Design review of the part built by this model. Coordinates are the model's own, in mm. A direction names the side the tool comes from. Coordinates: 2 decimals unless noted, no trailing zeros. Loops run counter-clockwise (first coordinate to the right, second up) from the corner with the lowest first, then second, coordinate; pieces in that order, holes last. Notation, with made-up numbers: (27, -15) - (62, -15) arc R15 ccw to (62, -4) - close; hole circle Ø10 at (-4.5, 44). An arc over 180 degrees is marked (long way). One line per question, with ' | ' between items.
from build123d import *

# Parameters (mm, degrees)
BOSS_EXTRUDE1_DEPTH  = 58.71
SKETCH4_R            = 4.8
CUT_EXTRUDE1_DEPTH   = 1
SKETCH5_R            = 4.8
CUT_EXTRUDE2_DEPTH   = 1
SKETCH6_W            = 19
SKETCH6_H            = 26
BOSS_EXTRUDE3_DEPTH  = 58.71
SKETCH7_W            = 58.71
SKETCH7_H            = 17
SKETCH7_H_2          = 19
BOSS_EXTRUDE4_DEPTH  = 57
BOSS_EXTRUDE5_DEPTH  = 3
CUT_EXTRUDE3_DEPTH   = 17
CUT_EXTRUDE4_START   = -19
CUT_EXTRUDE4_DEPTH   = 19
CUT_EXTRUDE5_DEPTH   = 4.632332886
SKETCH12_W           = 5
SKETCH12_H           = 5
BOSS_EXTRUDE6_DEPTH  = 100
CHAMFER1_SIZE        = 3
SKETCH13_W           = 61.71
SKETCH13_H           = 17.5
BOSS_EXTRUDE7_DEPTH  = 17
SKETCH14_W           = 24.98
SKETCH14_H           = 2.38
SKETCH14_W_2         = 14.02
BOSS_EXTRUDE8_DEPTH  = 12.5
BOSS_EXTRUDE9_DEPTH  = 5
BOSS_EXTRUDE10_START = -5
BOSS_EXTRUDE10_DEPTH = 5


with BuildPart() as part:
    # Sketch3 → Boss-Extrude1 (new body)
    with BuildSketch(Plane.YZ):
        Polygon((0, 5), (0, 0), (17, 0), (81, 26), (100, 26), (100, 31), (81, 31), (17, 5), align=None)
    extrude(amount=BOSS_EXTRUDE1_DEPTH)

    # Sketch4 → Cut-Extrude1 (cut)
    with BuildSketch(Plane.XY.offset(31)):
        with Locations((12.75, 90.5)):
            Circle(SKETCH4_R)
        with Locations((47.2, 90.5)):
            Circle(SKETCH4_R)
    extrude(amount=-CUT_EXTRUDE1_DEPTH, mode=Mode.SUBTRACT)

    # Sketch5 → Cut-Extrude2 (cut)
    with BuildSketch(Plane.XY.offset(5)):
        with Locations((21.94, 8.5)):
            Circle(SKETCH5_R)
        with Locations((36.94, 8.5)):
            Circle(SKETCH5_R)
    extrude(amount=-CUT_EXTRUDE2_DEPTH, mode=Mode.SUBTRACT)

    # Sketch6 → Boss-Extrude3 (add)
    with BuildSketch(Plane.YZ.offset(58.71)):
        with Locations((90.5, 13)):
            Rectangle(SKETCH6_W, SKETCH6_H)
    extrude(amount=-BOSS_EXTRUDE3_DEPTH)

    # Sketch7 → Boss-Extrude4 (add)
    with BuildSketch(Plane(origin=(0, 0, 0), x_dir=(1, 0, 0), z_dir=(0, 0, -1))):
        with Locations((29.355, -8.5)):
            Rectangle(SKETCH7_W, SKETCH7_H)
        with Locations((29.355, -90.5)):
            Rectangle(SKETCH7_W, SKETCH7_H_2)
    extrude(amount=BOSS_EXTRUDE4_DEPTH)

    # Sketch8 → Boss-Extrude5 (add)
    with BuildSketch(Plane.YZ.offset(58.71)):
        Polygon((100, 31), (81, 31), (17, 5), (0, 5), (0, -57), (17, -57), (17, 0), (81, 26), (81, -57), (100, -57), align=None)
    extrude(amount=BOSS_EXTRUDE5_DEPTH)

    # Sketch9 → Cut-Extrude3 (cut)
    with BuildSketch(Plane.XZ):
        with BuildLine():
            Line((15, -2.5), (46.71, -2.5))
            ThreePointArc((46.71, -2.5), (53.781067812, -5.428932188), (56.71, -12.5))
            Line((56.71, -12.5), (56.71, -42))
            ThreePointArc((56.71, -42), (53.781067812, -49.071067812), (46.71, -52))
            Line((46.71, -52), (15, -52))
            ThreePointArc((15, -52), (7.928932188, -49.071067812), (5, -42))
            Line((5, -42), (5, -12.5))
            ThreePointArc((5, -12.5), (7.928932188, -5.428932188), (15, -2.5))
        make_face()
    extrude(amount=-CUT_EXTRUDE3_DEPTH, mode=Mode.SUBTRACT)

    # Sketch10 → Cut-Extrude4 (cut)
    with BuildSketch(Plane(origin=(0, 100, 0), x_dir=(-1, 0, 0), z_dir=(0, 1, 0)).offset(CUT_EXTRUDE4_START)):
        with BuildLine():
            Line((-46.71, 23.5), (-15, 23.5))
            ThreePointArc((-15, 23.5), (-7.928932188, 20.571067812), (-5, 13.5))
            Line((-5, 13.5), (-5, -42))
            ThreePointArc((-5, -42), (-7.928932188, -49.071067812), (-15, -52))
            Line((-15, -52), (-46.71, -52))
            ThreePointArc((-46.71, -52), (-53.781067812, -49.071067812), (-56.71, -42))
            Line((-56.71, -42), (-56.71, 13.5))
            ThreePointArc((-56.71, 13.5), (-53.781067812, 20.571067812), (-46.71, 23.5))
        make_face()
    extrude(amount=CUT_EXTRUDE4_DEPTH, mode=Mode.SUBTRACT)

    # Sketch11 → Cut-Extrude5 (cut)
    with BuildSketch(Plane(origin=(0, 0.664710813, -1.636211232), x_dir=(1, 0, 0), z_dir=(0, -0.376377046955938, 0.9264665771223093))):
        with BuildLine():
            Line((17, 79.711481203), (44.71, 79.711481203))
            ThreePointArc((44.71, 79.711481203), (51.781067812, 76.782549014), (54.71, 69.711481203))
            Line((54.71, 69.711481203), (54.71, 34.631817046))
            ThreePointArc((54.71, 34.631817046), (51.781067812, 27.560749234), (44.71, 24.631817046))
            Line((44.71, 24.631817046), (17, 24.631817046))
            ThreePointArc((17, 24.631817046), (9.928932188, 27.560749234), (7, 34.631817046))
            Line((7, 34.631817046), (7, 69.711481203))
            ThreePointArc((7, 69.711481203), (9.928932188, 76.782549014), (17, 79.711481203))
        make_face()
    extrude(amount=-CUT_EXTRUDE5_DEPTH, mode=Mode.SUBTRACT)

    # Sketch12 → Boss-Extrude6 (add)
    with BuildSketch(Plane.XZ):
        with Locations((2.5, -54.5)):
            Rectangle(SKETCH12_W, SKETCH12_H)
        with Locations((59.21, -54.5)):
            Rectangle(SKETCH12_W, SKETCH12_H)
    extrude(amount=-BOSS_EXTRUDE6_DEPTH)

    # Chamfer1
    chamfer1_edges = [part.edges().sort_by_distance(p)[0] for p in [
        (2.5, 17, -52),
        (2.5, 81, -52),
        (59.21, 81, -52),
        (59.21, 17, -52),
    ]]
    chamfer(chamfer1_edges, length=CHAMFER1_SIZE)

    # Sketch13 → Boss-Extrude7 (add)
    with BuildSketch(Plane.XZ):
        with Locations((30.855, -3.75)):
            Rectangle(SKETCH13_W, SKETCH13_H)
    extrude(amount=-BOSS_EXTRUDE7_DEPTH)

    # Sketch14 → Boss-Extrude8 (add)
    with BuildSketch(Plane.XZ):
        with Locations((12.49, -11.31)):
            Rectangle(SKETCH14_W, SKETCH14_H)
        with Locations((54.7, -11.31)):
            Rectangle(SKETCH14_W_2, SKETCH14_H)
    extrude(amount=BOSS_EXTRUDE8_DEPTH)

    # Sketch15 → Boss-Extrude9 (add)
    with BuildSketch(Plane(origin=(0, 0, 0), x_dir=(0, -1, 0), z_dir=(-1, 0, 0))):
        with BuildLine():
            Line((0, -12.5), (12.5, -12.5))
            ThreePointArc((12.5, -12.5), (4.446217859, -15.360002914), (0, -22.6589186))
            Line((0, -22.6589186), (0, -12.5))
        make_face()
    extrude(amount=-BOSS_EXTRUDE9_DEPTH)

    # Sketch16 → Boss-Extrude10 (add)
    with BuildSketch(Plane.YZ.offset(61.71).offset(BOSS_EXTRUDE10_START)):
        with BuildLine():
            Line((-12.5, -12.5), (0, -12.5))
            Line((0, -12.5), (0, -22.6589186))
            ThreePointArc((0, -22.6589186), (-4.446217859, -15.360002914), (-12.5, -12.5))
        make_face()
    extrude(amount=BOSS_EXTRUDE10_DEPTH)


solid = part.part
Q1. Draft analysis for pull direction X (two halves, no side actions). For faces 1 (the flat face through (61.71, 82, -13)), 2 (the flat face through (33, 0, -52.5)), 3 (the flat face through (31, 90, 23.5)), state which applies: +X half, -X half, draft (parallel to the pull), parting line (faces both ways), or undercut.
Returned:
face 1: +X half | face 2: draft | face 3: undercut
Q2. To check wall thickness, follow line 1 along Y through (x, z) = (56, -53); line 2 along Y through (x, z) = (47.2, 30.35); line 3 along Z through (x, y) = (17, 8). State the ranges of each line that lie inside material, in increasing order.
Returned:
line 1: y = 0 to 17, 81 to 100 | line 2: y = 79.4 to 85.7, 95.3 to 100 | line 3: z = -57 to -52, -12.5 to 5
Q3. Take a section at C-C (y = 90.5). Give the boundary of the cut face in (x, z).
Returned:
outline: (0, -57) - (61.71, -57) - (61.71, 31) - (52, 31) - (52, 30) - (42.4, 30) - (42.4, 31) - (17.55, 31) - (17.55, 30) - (7.95, 30) - (7.95, 31) - (0, 31) - close; hole (5, -42) arc R10 ccw to (15, -52) - (46.71, -52) arc R10 ccw to (56.71, -42) - (56.71, 13.5) arc R10 ccw to (46.71, 23.5) - (15, 23.5) arc R10 ccw to (5, 13.5) - close
Q4. Take a section at A-A (x = 40). Give the boundary of the cut face in (y, z), plus the area to 3 significant figures.
Returned:
outline: (0, -57) - (17, -57) - (17, -52) - (0, -52) - close; (0, -12.5) - (17, -12.5) - (17, 0) - (25.23, 3.34) - (23.49, 7.63) - (17, 5) - (0, 5) - close; (74.51, 28.37) - (76.26, 24.07) - (81, 26) - (81, 23.5) - (100, 23.5) - (100, 31) - (81, 31) - close; (81, -57) - (100, -57) - (100, -52) - (81, -52) - close | area: 685 mm²
Q5. Take a section at D-D (y = 42). Give the boundary of the cut face in (x, z), plus the area to 3 significant figures.
Returned:
outline: (0, -57) - (5, -57) - (5, -52) - (0, -52) - close; (0, 10.16) - (7, 10.16) - (7, 15.16) - (0, 15.16) - close; (54.71, 10.16) - (61.71, 10.16) - (61.71, 15.16) - (54.71, 15.16) - close; (56.71, -57) - (61.71, -57) - (61.71, -52) - (56.71, -52) - close | area: 120 mm²
Q6. Take a section at B-B (z = -17.5). Give the boundary of the cut face in (x, y).
Returned:
outline: (0, -2.37) - (5, -2.37) - (5, 17) - (0, 17) - close; (0, 81) - (5, 81) - (5, 100) - (0, 100) - close; (56.71, -2.37) - (61.71, -2.37) - (61.71, 17) - (56.71, 17) - close; (56.71, 81) - (61.71, 81) - (61.71, 100) - (56.71, 100) - close
Q7. For pin 1 (12 mm diameter, centred on x = 19.5, z = 12, fed in from -Y); pin 2 (14 mm diameter, centred on x = 25.5, z = -1.5, fed in from -Y); pin 3 (5 mm diameter, centred on x = 13.5, y = 92.5, fed in from +Z); pin 4 (6 mm diameter, centred on x = 16, z = 11.5, fed in from +Y), all flat-tipped, find the tip position at first contact; note any pin that passes through.
Returned:
pin 1: stops at y = 19.46 | pin 2: stops at y = 0 | pin 3: stops at z = 30 | pin 4: passes through
Q8. Tool access review of faces 4 (the flat face through (47.69, -6, -11)), 5 (the flat face through (30.661, 75.374, 26.25)), 6 (the flat face through (3, 49, 13)), 7 (the flat face through (31.049, 24.345, 5.519)), 8 (the flat face through (56.71, 49, -54)): name each direction out of +Z, -Z, +X, -X, +Y, -Y from which nothing blocks a thin tool from reaching the whole face with its end or side.
Returned:
face 4: +Z, -Z, -Y | face 5: -Z, -Y | face 6: +X, -X | face 7: +Z, +Y | face 8: -Z
